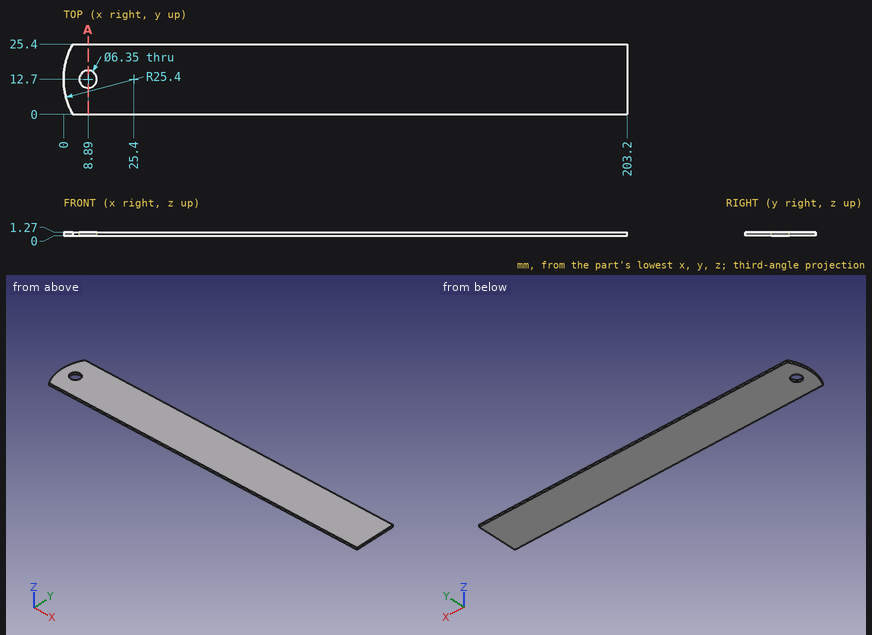
Design review of the part shown in the three views and the two pictorial views. Dimensions are in mm from the part's minimum x, y and z. Coordinates: 2 decimals unless noted, no trailing zeros. Order: outer loops, then holes, each group sorted by start corner. A loop starts at its lowest first (then second) coordinate and runs counter-clockwise, first axis right, second up.
1) Wall thickness on line 1 along Y through (x, z) = (8.89, 0.8) (3 decimals); line 2 along X through (y, z) = (11, 0.9); line 3 along X through (y, z) = (18.5, 0.3): over which ranges is each line inside the solid? List them lowest first.
2) Take a section at A-A, the plane x = 8.89. Give the boundary of the cut face in (y, z) (3 decimals), and give its area (3 significant figures).
3) Clearance check with a flat-ended pin moving along its axis: pin 1 (5.5 mm diameter, centred on x = 8.89, y = 12.7, fed in from -Z). State where the tip first meets the part, or that it passes through.
Returned:
1. line 1: y = 0 to 9.525, 15.875 to 25.4
1. line 2: x = 0.06 to 6.21, 11.57 to 203.2
1. line 3: x = 0.67 to 203.2
2. outline: (0, 0) - (9.525, 0) - (9.525, 1.27) - (0, 1.27) - close; (15.875, 0) - (25.4, 0) - (25.4, 1.27) - (15.875, 1.27) - close
2. area: 24.2 mm2
3. pin 1: passes through
